Design review of the part built by this model. Coordinates are the model's own, in mm. Coordinates: 2 decimals unless noted, no trailing zeros. Loops run counter-clockwise (first coordinate to the right, second up) from the corner with the lowest first, then second, coordinate; pieces in that order, holes last. Notation, with made-up numbers: M -31,-20.5 L 14,-20.5 A23 ccw 14,-7.5 Z; hole C 46,-36.75 d11. An arc over 180 degrees is marked long. Put each result on its own line as item: value. Start each with the question number.
(1) For probe 1 along Z at (x, y) = (-61, 5); probe 2 along Z at (x, y) = (-22, 7.5); probe 3 along Y at (x, z) = (-59, 78), list the stretches that pass through material, from the lowest coordinate up. Write a range as [from, to].
(2) Take a section at B-B, the plane z = 31.5. Give the boundary of the cut face in (x, y), then the cut area to 3 significant figures.
(3) Take a section at C-C, the plane x = -22. Give the boundary of the cut face in (y, z).
(4) Take a section at A-A, the plane y = 8.5. Give the boundary of the cut face in (x, z).
```python
from build123d import *

# Parameters (mm, degrees)
SKETCH1_W           = 68.58
SKETCH1_H           = 88.9
BOSS_EXTRUDE1_DEPTH = 2.54
SKETCH2_W           = 68.58
SKETCH2_H           = 5.08
BOSS_EXTRUDE2_DEPTH = 7.62
SKETCH3_W           = 68.58
SKETCH3_H           = 3.048
BOSS_EXTRUDE3_DEPTH = 6.35
SKETCH4_W           = 68.58
SKETCH4_H           = 3.048
BOSS_EXTRUDE4_DEPTH = 6.35
SKETCH5_W           = 68.58
SKETCH5_H           = 26.416
SKETCH5_H_2         = 21.59
SKETCH5_H_3         = 7.874
BOSS_EXTRUDE5_DEPTH = 7.62
SKETCH6_W           = 4.572
SKETCH6_H           = 1.27
SKETCH6_W_2         = 3.048
CUT_EXTRUDE1_DEPTH  = 113.737092388


with BuildPart() as part:
    # Sketch1 → Boss-Extrude1 (new body)
    with BuildSketch(Plane(origin=(0, 0, 0), x_dir=(-1, 0, 0), z_dir=(0, 1, 0))):
        with Locations((34.29, 44.45)):
            Rectangle(SKETCH1_W, SKETCH1_H)
    extrude(amount=BOSS_EXTRUDE1_DEPTH)

    # Sketch2 → Boss-Extrude2 (add)
    with BuildSketch(Plane(origin=(0, 2.54, 0), x_dir=(-1, 0, 0), z_dir=(0, 1, 0))):
        with Locations((34.29, 67.056)):
            Rectangle(SKETCH2_W, SKETCH2_H)
        with Locations((34.29, 28.956)):
            Rectangle(SKETCH2_W, SKETCH2_H)
    extrude(amount=BOSS_EXTRUDE2_DEPTH)

    # Sketch3 → Boss-Extrude3 (add)
    with BuildSketch(Plane.XY.offset(31.496)):
        with Locations((-34.29, 8.636)):
            Rectangle(SKETCH3_W, SKETCH3_H)
    extrude(amount=BOSS_EXTRUDE3_DEPTH)

    # Sketch4 → Boss-Extrude4 (add)
    with BuildSketch(Plane.XY.offset(69.596)):
        with Locations((-34.29, 8.636)):
            Rectangle(SKETCH4_W, SKETCH4_H)
    extrude(amount=BOSS_EXTRUDE4_DEPTH)

    # Sketch5 → Boss-Extrude5 (add)
    with BuildSketch(Plane(origin=(0, 2.54, 0), x_dir=(-1, 0, 0), z_dir=(0, 1, 0))):
        with Locations((34.29, 13.208)):
            Rectangle(SKETCH5_W, SKETCH5_H)
        with Locations((34.29, 53.721)):
            Rectangle(SKETCH5_W, SKETCH5_H_2)
        with Locations((34.29, 84.963)):
            Rectangle(SKETCH5_W, SKETCH5_H_3)
    extrude(amount=BOSS_EXTRUDE5_DEPTH)

    # Sketch6 → Cut-Extrude1 (cut, through all)
    with BuildSketch(Plane.YZ):
        with Locations((4.826, 68.961)):
            Rectangle(SKETCH6_W, SKETCH6_H)
        with Locations((4.826, 30.861)):
            Rectangle(SKETCH6_W, SKETCH6_H)
        with Locations((8.636, 37.211)):
            Rectangle(SKETCH6_W_2, SKETCH6_H)
        with Locations((8.636, 75.311)):
            Rectangle(SKETCH6_W_2, SKETCH6_H)
    extrude(amount=-CUT_EXTRUDE1_DEPTH, mode=Mode.SUBTRACT)


solid = part.part
```
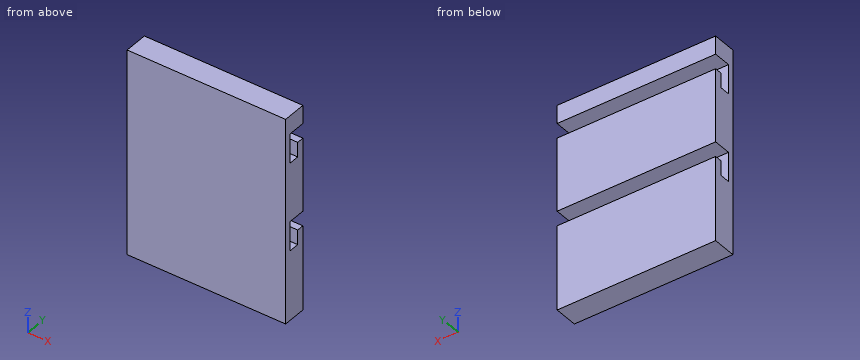
Computed values:
1. probe 1: z = [0, 30.23], [42.93, 68.33], [81.03, 88.9]
1. probe 2: z = [0, 36.58], [42.93, 74.68], [81.03, 88.9]
1. probe 3: y = [0, 2.54]
2. outline: M -68.58,0 L 0,0 L 0,2.54 L -68.58,2.54 Z; M -68.58,7.11 L 0,7.11 L 0,10.16 L -68.58,10.16 Z
2. area: 383 mm^2
3. outline: M 0,0 L 10.16,0 L 10.16,36.58 L 7.11,36.58 L 7.11,30.23 L 2.54,30.23 L 2.54,42.93 L 10.16,42.93 L 10.16,74.68 L 7.11,74.68 L 7.11,68.33 L 2.54,68.33 L 2.54,81.03 L 10.16,81.03 L 10.16,88.9 L 0,88.9 Z
4. outline: M -68.58,0 L 0,0 L 0,36.58 L -68.58,36.58 Z; M -68.58,42.93 L 0,42.93 L 0,74.68 L -68.58,74.68 Z; M -68.58,81.03 L 0,81.03 L 0,88.9 L -68.58,88.9 Z
